Here's how the part is built. I have some questions about the finished solid (model axes, mm). A direction names the side the tool comes from. Coordinates: 2 decimals unless noted, no trailing zeros. Write each loop counter-clockwise with the first axis right and the second up, starting at its lowest first coordinate (ties: lowest second). Pieces come first, ordered by that corner, then holes.
Item 1: If I drill on line 1 (Z direction, x = 2.5, y = -5); line 2 (Y direction, x = -5.75, z = 23); line 3 (X direction, y = 9, z = 20), over which ranges is the centre line in solid material (lowest first)?
Item 2: I'm going to push flat-ended pins straight in: pin 1 Ø2 at (y, z) = (9, 21) entering from -X; pin 2 Ø2 at (y, z) = (7.5, 14.5) entering from -X; pin 3 Ø4.5 at (y, z) = (9.5, 22) entering from +X. Where does each tip first touch, or does it pass through?
Item 3: If we section it at A-A (x = 0): Please give me the cut outline in (y, z), then the cut area to 3 significant figures.
Item 4: If we section it at D-D (x = -9.25): Please give me the cut outline in (y, z), then the cut area to 3 significant figures.
Item 5: If we section it at C-C (z = 7.5): Please give me the cut outline in (x, y).
Item 6: For faces 1 (the face through (0, -1, 0)), 2 (the face through (1.6, 10, 21)), which set-ups out of +Z, -Z, +X, -X, +Y, -Y let a thin tool reach every point of the face, with its end or its side?
Item 7: If we section it at B-B (y = 6.25): Please give me the cut outline in (x, z).
Item 8: We'd pull the mould along Z, two halves only. Please class faces 3 (the face through (0, 10, 17.4)), 4 (the face through (0.04, 9.97, 25.38)), 5 (the face through (9.965, 9.765, 12.164)), 6 (the face through (11.9, -11.43, 1.52)): +Z half, -Z half, draft (parallel to the pull), parting line (faces both ways), or undercut.
from build123d import *

# Parameters (mm, degrees)
SKETCH_W        = 25
SKETCH_H        = 24
PAD_DEPTH       = 3
PAD001_DEPTH    = 24
POCKET_DEPTH    = 20
POCKET001_DEPTH = 27
POCKET002_DEPTH = 4
FILLET_R        = 2
FILLET001_R     = 2


with BuildPart() as part:
    # Sketch → Pad (new body)
    with BuildSketch(Plane.XY):
        Rectangle(SKETCH_W, SKETCH_H)
    extrude(amount=PAD_DEPTH)

    # Sketch001 → Pad001 (new body)
    with BuildSketch(Plane(origin=(0, 12, 0), x_dir=(-1, 0, 0), z_dir=(0, 1, 0))):
        with BuildLine():
            Line((12.5, 3), (7.5, 21.074721))
            ThreePointArc((7.5, 21.074721), (0, 26.781675), (-7.5, 21.074721))
            Line((-7.5, 21.074721), (-12.5, 3))
            Line((12.5, 3), (-12.5, 3))
        make_face()
    extrude(amount=-PAD001_DEPTH)

    # Sketch002 → Pocket (cut)
    with BuildSketch(Plane.XZ.offset(12)):
        Polygon((10.5, 3), (-10.5, 3), (-7.733706, 13), (-15, 13), (-15, 26.781675), (15, 26.781675), (15, 13), (7.733706, 13), align=None)
    extrude(amount=-POCKET_DEPTH, mode=Mode.SUBTRACT)

    # Sketch003 → Pocket001 (cut)
    with BuildSketch(Plane.YZ.offset(12.5)):
        with BuildLine():
            ThreePointArc((-1.99997, 3), (8, 13), (-1.99997, 23))
            Line((-12, 23), (-1.99997, 23))
            Line((-12, 3), (-12, 23))
            Line((-1.99997, 3), (-12, 3))
        make_face()
    extrude(amount=-POCKET001_DEPTH, mode=Mode.SUBTRACT)

    # Sketch004 → Pocket002 (cut)
    with BuildSketch(Plane.XZ.offset(-8)):
        with BuildLine():
            ThreePointArc((1.6, 23.781675), (0, 25.381675), (-1.6, 23.781675))
            Line((-1.6, 23.781675), (-1.6, 19))
            ThreePointArc((-1.6, 19), (0, 17.4), (1.6, 19))
            Line((1.6, 23.781675), (1.6, 19))
        make_face()
    extrude(amount=-POCKET002_DEPTH, mode=Mode.SUBTRACT)

    # Fillet
    fillet_edges = [part.edges().sort_by_distance(p)[0] for p in [
        (12.5, -12, 1.5),
        (-12.5, -12, 1.5),
    ]]
    fillet(fillet_edges, radius=FILLET_R)

    # Fillet001
    fillet001_edges = [part.edges().sort_by_distance(p)[0] for p in [
        (0, 12, 0),
    ]]
    fillet(fillet001_edges, radius=FILLET001_R)


solid = part.part
Answer list:
1. line 1: z = 0 to 3
1. line 2: y = 8 to 12
1. line 3: x = -7.8 to -1.6, 1.6 to 7.8
2. pin 1: stops at x = -7.8
2. pin 2: stops at x = -9.56
2. pin 3: stops at x = 7.87
3. outline: (-12, 0) - (10, 0) arc R2 ccw to (12, 2) - (12, 17.4) - (8, 17.4) - (8, 3) - (-12, 3) - close; (8, 25.38) - (12, 25.38) - (12, 26.78) - (8, 26.78) - close
3. area: 134 mm2
4. outline: (-12, 0) - (10, 0) arc R2 ccw to (12, 2) - (12, 14.75) - (8, 14.75) - (8, 13) arc R10 cw to (6.36, 7.52) - (8, 7.52) - (8, 3) - (-12, 3) - close
4. area: 121 mm2
5. outline: (-11.26, 6.35) - (-9.26, 6.35) - (-9.26, 8) - (9.26, 8) - (9.26, 6.35) - (11.26, 6.35) - (11.26, 12) - (-11.26, 12) - close
6. face 1: -Z, +X, -X, +Y, -Y
6. face 2: +Y, -Y
7. outline: (-12.5, 0) - (12.5, 0) - (12.5, 3) - (11.3, 7.35) - (9.3, 7.35) - (10.5, 3) - (-10.5, 3) - (-9.3, 7.35) - (-11.3, 7.35) - (-12.5, 3) - close
8. face 3: undercut
8. face 4: undercut
8. face 5: +Z half
8. face 6: draft
